Autodesk Inventor part; units mm, degrees
ref_plane "Work Plane1" through (0, 0, 22.225) normal (-1, 0, 0) x (0, 0, 1)
sketch "Sketch1" plane through (0, 0, 0) normal (0, 1, 0) x (-1, 0, 0)
  line L0 (7.9375, 22.225) -> (-7.9375, 22.225)
  line L1 (-7.9375, 22.225) -> (-7.9375, -22.225)
  line L2 (-7.9375, -22.225) -> (7.9375, -22.225)
  line L3 (7.9375, -22.225) -> (7.9375, 22.225)
  line L4 (7.9375, 22.225) -> (-7.9375, -22.225) construction
  line L5 (-7.9375, 22.225) -> (7.9375, -22.225) construction
  point P0 (0, 0)
  point P1 (-50.8, 0)
  dimension "d0" = 15.875
  dimension "d1" = 44.45
extrude "Base" add sketch "Sketch1" along normal blind 4.7625
sketch "Sketch2" plane through (7.9375, 0, 22.225) normal (1, 0, 0) x (0, 0, -1)
  line L0 (0, 0) -> (0, 4.7625)
  line L1 (0, 4.7625) -> (10.2968, 32.9347)
  line L2 (0, 4.7625) -> (44.45, 4.7625)
  line L3 (34.1532, 32.9347) -> (44.45, 4.7625)
  line L4 (0, 0) -> (44.45, 0)
  arc A0 (34.1532, 32.9347) -> (10.2968, 32.9347) centre (22.225, 28.575) ccw
  line L5 (0, 0) -> (44.45, 0)
  line L6 (44.45, 0) -> (44.45, 4.7625)
  line L7 (0, 4.7625) -> (44.45, 4.7625)
  line L8 (0, 0) -> (0, 4.7625)
  point P0 (22.225, 0)
  point P1 (22.225, 41.275)
  dimension "d10" = 12.7
  dimension "d12" = 41.275
extrude "Vertical 1" add sketch "Sketch2" along normal blind 4.7625
sketch "Sketch5" plane through (-7.9375, 0, -22.225) normal (-1, 0, 0) x (0, 0, 1)
  line L0 (44.45, 4.7625) -> (44.45, 0)
  line L1 (44.45, 0) -> (0, 0)
  line L2 (0, 0) -> (0, 4.7625)
  line L3 (0, 4.7625) -> (10.2968, 32.9347)
  arc A0 (34.1532, 32.9347) -> (10.2968, 32.9347) centre (22.225, 28.575) ccw
  line L4 (34.1532, 32.9347) -> (44.45, 4.7625)
extrude "Vertical 2" add sketch "Sketch5" along normal blind 4.7625
sketch "Sketch6" plane through (12.7, 0, 22.225) normal (1, 0, 0) x (0, 0, -1)
  line L0 (22.225, 0) -> (22.225, 41.275) construction
  arc A0 (34.1532, 32.9347) -> (10.2968, 32.9347) centre (22.225, 28.575) ccw
  circle A1 centre (22.225, 31.75) radius 6.35
  dimension "d29" = 12.7
  dimension "d30" = 9.525
extrude "Extrusion8" cut sketch "Sketch6" against normal through all
fillet "Fillet2" radius 3.175 6 edges at (-12.7, 0, 0) (-12.7, 2.3813, -22.225) (12.7, 2.3813, -22.225) (12.7, 2.3813, 22.225) (12.7, 0, 0) (-12.7, 2.3813, 22.225)
chamfer "Chamfer2" distance 1.27 angle 45 2 edges at (-7.9375, 4.7625, 0) (7.9375, 4.7625, 0)
ref_plane "Work Plane2" through (0, 31.75, 0) normal (0, 1, 0) x (-1, 0, 0)
ref_plane "Work Plane1" through (0, 0, 22.225) normal (-1, 0, 0) x (0, 0, 1)
equation "\"BendRadius\" = Thickness"
equation "\"BendReliefWidth\" = Thickness"
equation "\"BendReliefDepth\" = 0.5 * Thickness"
equation "\"CornerReliefSize\" = 4 * Thickness"
equation "\"MinimumRemnant\" = 2 * Thickness"
equation "\"TransitionRadius\" = BendRadius"
equation "\"JacobiRadiusSize\" = BendRadius"
equation "\"GapSize\" = Thickness"
properties part number "0.5 in Rod End Bracket (Rough)"
Can you work these out from the model? Positions are in its coordinate system, mm. A direction names the side the tool comes from. Give positions to 0.01 mm unless a question says otherwise; leave off trailing zeros. Loops run counter-clockwise (first coordinate to the right, second up) from the corner with the lowest first, then second, coordinate; pieces in that order, holes last. Notation, with made-up numbers: (-34, 17.25) -> (-8, 17.25) arc R17 ccw to (-8, 22.25) -> close; hole circle Ø3 at (37, 4). An arc over 180 degrees is marked (long way). Return JSON: item names as keys, results as strings.
Q1. I want a section at A-A, the plane z = 0. Count the separate pieces of the cut face and the enclosed holes in it, then the cut area to 3 significant figures.
Checks:
{"separate pieces": "3", "enclosed holes": "0", "area": "345 mm2"}
Q2. I want a section at B-B, the plane y = 31.75. List the corners of the cut face in (x, z) for me, then the cut area to 3 significant figures.
Checks:
{"outline": "(-12.7, -12.36) -> (-7.94, -12.36) -> (-7.94, -6.35) -> (-12.7, -6.35) -> close; (-12.7, 6.35) -> (-7.94, 6.35) -> (-7.94, 12.36) -> (-12.7, 12.36) -> close; (7.94, -12.36) -> (12.7, -12.36) -> (12.7, -6.35) -> (7.94, -6.35) -> close; (7.94, 6.35) -> (12.7, 6.35) -> (12.7, 12.36) -> (7.94, 12.36) -> close", "area": "115 mm2"}
Q3. I want a section at D-D, the plane y = 17.5. List the corners of the cut face in (x, z) for me, then the cut area to 3 significant figures.
Checks:
{"outline": "(-12.7, -17.57) -> (-7.94, -17.57) -> (-7.94, 17.57) -> (-12.7, 17.57) -> close; (7.94, -17.57) -> (12.7, -17.57) -> (12.7, 17.57) -> (7.94, 17.57) -> close", "area": "335 mm2"}
Q4. On a 3-axis mill with a long thin cutter (end or side, diameter ignored), from which of +Z, -Z, +X, -X, +Y, -Y can I reach the whole of each face in a straight line? I mean faces 1 (the face through (-10.31, 18.65, -17.15)), 2 (the face through (7.311, 5.406, -0.311)). Say none if no direction works.
Checks:
{"face 1": "-Z, +X, -X, +Y", "face 2": "+Z, -Z, +Y"}
Q5. We'd pull the mould along X, two halves only. Please class faces 3 (the face through (12.106, 5.324, 20.9)), 4 (the face through (-7.311, 5.406, 0.311)), 5 (the face through (0, 0, 0)), 6 (the face through (7.938, 20, 0)): released by +X, released by -X, zero draft, split by the parting line, or undercut.
Checks:
{"face 3": "released by +X", "face 4": "undercut", "face 5": "zero draft", "face 6": "undercut"}
Q6. For pin 1 Ø1 at (x, z) = (6, 7) entering from +Y; pin 2 Ø6 at (x, y) = (-7.5, 21.5) entering from -Z; pin 3 Ø5 at (x, y) = (-7.5, 20.5) entering from +Z; pin 4 Ø8 at (x, y) = (2, 29.5) entering from -Z, each with a flat end and sliding along its axis, tell me the tip position at first contact or that it passes through.
Checks:
{"pin 1": "stops at y = 4.76", "pin 2": "stops at z = -17.19", "pin 3": "stops at z = 17.37", "pin 4": "passes through"}
Q7. I need wall thicknesses on probe 1 along X at (y, z) = (12.5, 2.5); probe 2 along Y at (x, z) = (9.1, 0); probe 3 along Y at (x, z) = (-10.75, -4). Which ranges of each line are inside material? Lowest first, please.
Checks:
{"probe 1": "x = -12.7 to -7.94, 7.94 to 12.7", "probe 2": "y = 0 to 25.4, 38.1 to 41.27", "probe 3": "y = 0.25 to 26.82, 36.68 to 40.63"}
